```python
from build123d import *

# Parameters (mm, degrees)
SKETCH1_W                 = 17.5
SKETCH1_H                 = 10
BASE_FLANGE1_DEPTH        = 1.6
F_4_CLEARANCE_HOLE1_D     = 3.2639
F_4_CLEARANCE_HOLE1_DEPTH = 1.6
F_4_CLEARANCE_HOLE1_TIP   = 0.980574487
EDGE_FLANGE1_DEPTH        = 17.5
SKETCH20_R                = 4
CUT_EXTRUDE1_DEPTH        = 1.6


# Sheet-metal steps are written as plain solids
with BuildPart() as part:
    # Sketch1 → Base-Flange1 (new body)
    with BuildSketch(Plane(origin=(0, 0, 0), x_dir=(1, 0, 0), z_dir=(0, 1, 0))):
        with Locations((-14.536713287, 16.32983683)):
            Rectangle(SKETCH1_W, SKETCH1_H)
    extrude(amount=-BASE_FLANGE1_DEPTH)

    # #4 Clearance Hole1
    with Locations(Plane.XZ.offset(1.6)):
        with Locations((-9.786713287, -16.32983683), (-19.286713287, -16.32983683)):
            Hole(F_4_CLEARANCE_HOLE1_D / 2, depth=F_4_CLEARANCE_HOLE1_DEPTH)
            with Locations((0, 0, -(F_4_CLEARANCE_HOLE1_DEPTH + F_4_CLEARANCE_HOLE1_TIP / 2))):  # 118° drill point
                Cone(0, F_4_CLEARANCE_HOLE1_D / 2, F_4_CLEARANCE_HOLE1_TIP, mode=Mode.SUBTRACT)

    # Edge-Flange1 section (across the edge) → Edge-Flange1 (add)
    with BuildSketch(Plane(origin=(-23.286713287, -1.6, -25.06643683), x_dir=(0, 0, 1), z_dir=(1, 0, 0))):
        with BuildLine():
            Line((-1.6, 0.7366), (-1.6, 24.4))
            Line((-1.6, 24.4), (0, 24.4))
            Line((0, 24.4), (0, 0.7366))
            ThreePointArc((0, 0.7366), (0.215745145, 0.215745145), (0.7366, 0))
            Line((0.7366, 0), (3.7366, 0))
            Line((3.7366, 0), (3.7366, -1.6))
            Line((3.7366, -1.6), (0.7366, -1.6))
            ThreePointArc((0.7366, -1.6), (-0.915625705, -0.915625705), (-1.6, 0.7366))
        make_face()
    extrude(amount=EDGE_FLANGE1_DEPTH)

    # Sketch20 → Cut-Extrude1 (cut)
    with BuildSketch(Plane(origin=(0, 0, -26.66643683), x_dir=(-1, 0, 0), z_dir=(0, 0, -1))):
        with Locations(Location((14.536713287, -13, 0), (0, 0, 90))):
            Circle(SKETCH20_R)
    extrude(amount=-CUT_EXTRUDE1_DEPTH, mode=Mode.SUBTRACT)


solid = part.part
```
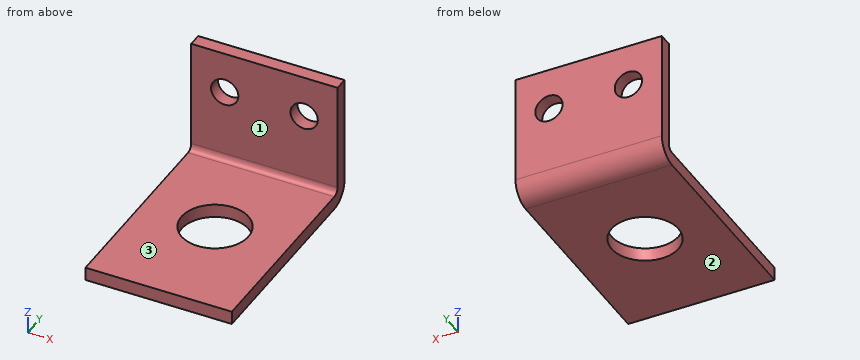
Geometry check sheet. Reference: the model listing, model coordinates, mm. Face numbers are marked on the shaded views. Round coordinates to 2 decimals unless told otherwise and drop trailing zeros. Write each loop counter-clockwise with the first axis right and the second up, starting at its lowest first coordinate (ties: lowest second). Pieces come first, ordered by that corner, then holes. Notation, with made-up numbers: (-23.75, 61.25) - (0.25, 61.25) arc R27 cw to (0.25, 87.25) - close; hole circle Ø1 at (-23, 37.25). An arc over 180 degrees is marked (long way). Write each question's results on one line, items separated by ' | '.
(1) Sectioned sample at C-C, the plane y = -15.75. Enter the section's corners in (x, z).
Computed:
outline: (-23.29, -26.67) - (-17.44, -26.67) - (-17.44, -25.07) - (-23.29, -25.07) - close; (-11.63, -26.67) - (-5.79, -26.67) - (-5.79, -25.07) - (-11.63, -25.07) - close
(2) Draft check along Z on the marked faces 1, 2 and 3. Enter one of: pulls with the +Z half, pulls with the -Z half, needs draft (parallel to the pull), parting line crosses it, or undercut.
Computed:
face 1: needs draft | face 2: pulls with the -Z half | face 3: pulls with the +Z half
(3) Sectioned sample at B-B, the plane x = -22. Enter the section's corners in (y, z).
Computed:
outline: (-26, -26.67) - (-2.34, -26.67) arc R2.34 ccw to (0, -24.33) - (0, -11.33) - (-1.6, -11.33) - (-1.6, -24.33) arc R0.74 cw to (-2.34, -25.07) - (-26, -25.07) - close
(4) Depth check by flat-ended pin: pin 1 Ø2 at (x, z) = (-9.79, -16.33) entering from -Y; pin 2 Ø2 at (x, z) = (-18, -13.5) entering from -Y; pin 3 Ø1.5 at (x, y) = (-7.5, -15.5) entering from +Z. Enter the tip coordinate at first touch or a pass-through.
Computed:
pin 1: passes through | pin 2: stops at y = -1.6 | pin 3: stops at z = -25.07
(5) Sectioned sample at D-D, the plane z = -18.5. Enter the section's corners in (x, y), plus the area to 3 significant figures.
Computed:
outline: (-23.29, -1.6) - (-5.79, -1.6) - (-5.79, 0) - (-23.29, 0) - close | area: 28.0 mm^2
(6) Sectioned sample at A-A, the plane y = -13. Enter the section's corners in (x, z).
Computed:
outline: (-23.29, -26.67) - (-18.54, -26.67) - (-18.54, -25.07) - (-23.29, -25.07) - close; (-10.54, -26.67) - (-5.79, -26.67) - (-5.79, -25.07) - (-10.54, -25.07) - close
(7) Thickness scan on probe 1 along X at (y, z) = (-1.5, -15.75); probe 2 along Z at (x, y) = (-22.5, -14); probe 3 along X at (y, z) = (-13, -25.7). Record the ranges inside material, lowest first. Write a range as from..to.
Computed:
probe 1: x = -23.29..-20.81, -17.76..-11.31, -8.26..-5.79 | probe 2: z = -26.67..-25.07 | probe 3: x = -23.29..-18.54, -10.54..-5.79
